Autodesk Inventor part; units mm, degrees
ref_plane "YZ Plane" through (0, 0, 0) normal (1, 0, 0) x (0, 1, 0)
ref_plane "XZ Plane" through (0, 0, 0) normal (0, 1, 0) x (-1, 0, 0)
ref_plane "XY Plane" through (0, 0, 0) normal (0, 0, 1) x (1, 0, 0)
sketch "Sketch1" plane through (0, 0, 0) normal (0, 1, 0) x (-1, 0, 0)
  circle A0 centre (0, 0) radius 50
  circle A1 centre (0, 0) radius 2.5527
  line L0 (1.4351, -2.1111) -> (-1.4351, -2.1111)
  dimension "d0" = 100
  dimension "d1" = 5.1054
  dimension "d2" = 2.8702
extrude "Extrusion1" add sketch "Sketch1" along normal blind 10 contours A0 | L0 A1 picked at (0.2983, -2.2043)
sketch "Sketch2" plane through (0, 10, 0) normal (0, 1, 0) x (1, 0, 0)
  circle A0 centre (0, 0) radius 45
  dimension "d5" = 90
extrude "Extrusion2" cut sketch "Sketch2" against normal blind 9
sketch "Sketch7" plane through (0, 1, 0) normal (0, 1, 0) x (1, 0, 0)
  circle A0 centre (0, 0) radius 45
extrude "Extrusion5" cut sketch "Sketch7" along normal blind 10
properties part number "Gearsp1"
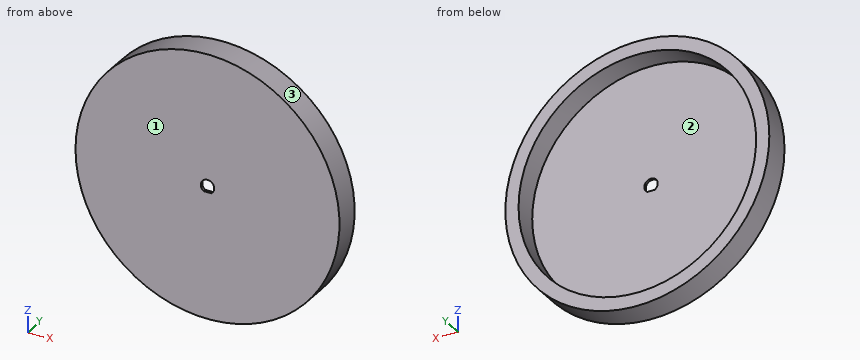
Verification items for the finished model (mm, model axes). Face numbers are marked on the shaded views. Give positions to 0.01 mm unless a question says otherwise; leave off trailing zeros. Order: outer loops, then holes, each group sorted by start corner. A loop starts at its lowest first (then second) coordinate and runs counter-clockwise, first axis right, second up. Notation, with made-up numbers: (-31, 34) -> (24, 34) arc R5 ccw to (24, 42) -> close; hole circle Ø7 at (-16.5, 77.5). An arc over 180 degrees is marked (long way). Answer as CSV lines item,"result".
Q1. Sectioned sample at A-A on x = 0. Record the cut outline in (y, z).
Solutions:
outline,"(0, -50) -> (10, -50) -> (10, -45) -> (1, -45) -> (1, -2.11) -> (0, -2.11) -> close; (0, 2.55) -> (1, 2.55) -> (1, 45) -> (10, 45) -> (10, 50) -> (0, 50) -> close"
Q2. Sectioned sample at C-C on y = 2.5. Record the cut outline in (x, z).
Solutions:
outline,"circle Ø100 at (0, 0); hole circle Ø90 at (0, 0)"
Q3. Sectioned sample at D-D on x = -34.5. Record the cut outline in (y, z), plus the area to 3 significant figures.
Solutions:
outline,"(0, -36.19) -> (10, -36.19) -> (10, -28.89) -> (1, -28.89) -> (1, 28.89) -> (10, 28.89) -> (10, 36.19) -> (0, 36.19) -> close"
area,"204 mm²"
Q4. Sectioned sample at B-B on z = 0. Record the cut outline in (x, y).
Solutions:
outline,"(-50, 0) -> (-2.55, 0) -> (-2.55, 1) -> (-45, 1) -> (-45, 10) -> (-50, 10) -> close; (2.55, 0) -> (50, 0) -> (50, 10) -> (45, 10) -> (45, 1) -> (2.55, 1) -> close"
Q5. Release check for a two-part mould opening along X. For the marked faces 1, 2 and 3 record: +X half, -X half, draft (parallel to the pull), parting line (faces both ways), or undercut.
Solutions:
face 1,"draft"
face 2,"undercut"
face 3,"parting line"
Q6. Depth check by flat-ended pin: pin 1 (2 mm diameter, centred on x = 29, y = 2, fed in from -Z); pin 2 (3 mm diameter, centred on x = -29, z = -22.5, fed in from +Y); pin 3 (1 mm diameter, centred on x = -31, y = 5, fed in from -Z). Enter the tip coordinate at first touch or a pass-through.
Solutions:
pin 1,"stops at z = -41.42"
pin 2,"stops at y = 1"
pin 3,"stops at z = -39.62"
Q7. Scan lines: probe 1 along Z at (x, y) = (0, 7.25); probe 2 along Y at (x, z) = (11, 2.5); probe 3 along Z at (x, y) = (-8, 8.25). Record each from-to range of solid material in increasing order.
Solutions:
probe 1,"z = -50 to -45, 45 to 50"
probe 2,"y = 0 to 1"
probe 3,"z = -49.36 to -44.28, 44.28 to 49.36"
